Part print with two shaded views. Sizes in mm from the minimum x, y, z corner. Coordinates: 2 decimals unless noted, no trailing zeros. Write each loop counter-clockwise with the first axis right and the second up, starting at its lowest first coordinate (ties: lowest second). Pieces come first, ordered by that corner, then holes.
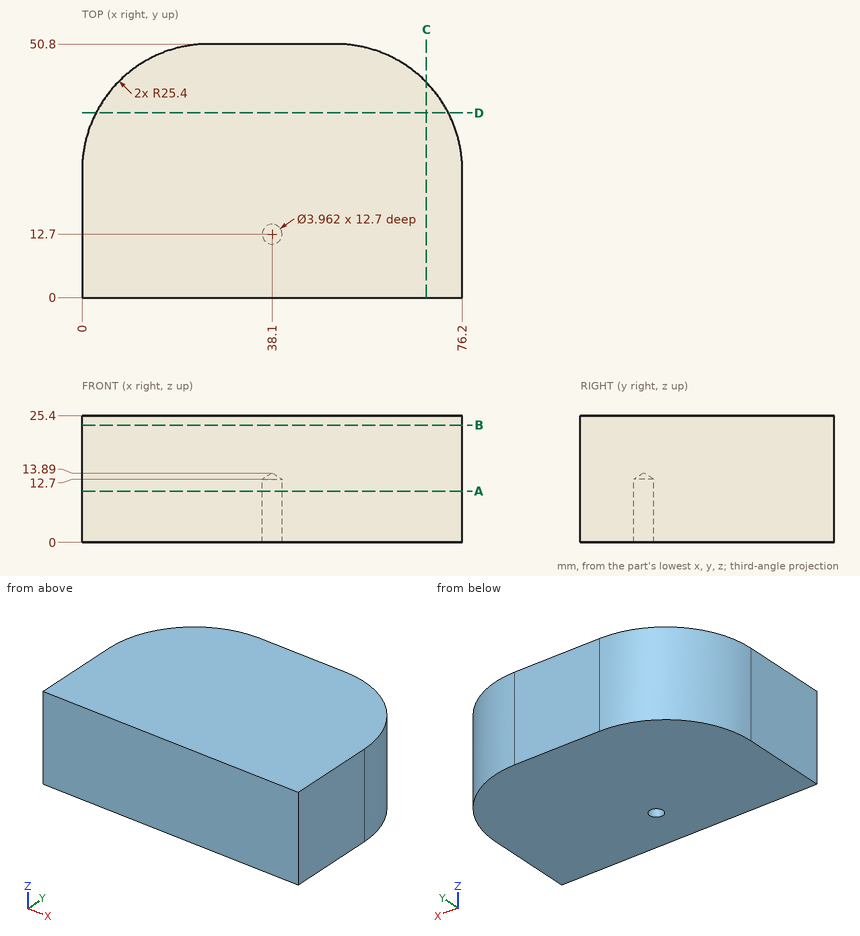
(1) Slice it at D-D, the plane y = 37. List the corners of the cut face in (x, z), and give its area (3 significant figures).
(2) Slice it at B-B, the plane z = 23.5. List the corners of the cut face in (x, y), and give its area (3 significant figures).
(3) Probe L1, parallel to X at y = 12.5, z = 8; L2, parallel to Y at x = 38.1, z = 6.75; L3, parallel to Y at x = 51, z = 15. List the from-to ranges inside material, lowest first.
(4) Slice it at C-C, the plane x = 69. List the corners of the cut face in (y, z).
(5) Slice it at A-A, the plane z = 10.25. List the corners of the cut face in (x, y).
(6) Flat gauge pins, fed straight in: P1, Ø2, axis at y = 44.5, z = 6.5, coming from the +X side; P2, Ø6, axis at y = 33, z = 16.5, coming from the +X side; P3, Ø3, axis at x = 38.1, y = 12.7, coming from the -Z side. Where does each tip first touch, or does it go through?
Results:
1. outline: (2.8, 0) - (73.4, 0) - (73.4, 25.4) - (2.8, 25.4) - close
1. area: 1,790 mm2
2. outline: (0, 0) - (76.2, 0) - (76.2, 25.4) arc R25.4 ccw to (50.8, 50.8) - (25.4, 50.8) arc R25.4 ccw to (0, 25.4) - close
2. area: 3,590 mm2
3. L1: x = 0 to 36.13, 40.07 to 76.2
3. L2: y = 0 to 10.72, 14.68 to 50.8
3. L3: y = 0 to 50.8
4. outline: (0, 0) - (43.12, 0) - (43.12, 25.4) - (0, 25.4) - close
5. outline: (0, 0) - (76.2, 0) - (76.2, 25.4) arc R25.4 ccw to (50.8, 50.8) - (25.4, 50.8) arc R25.4 ccw to (0, 25.4) - close; hole circle Ø3.96 at (38.1, 12.7)
6. P1: stops at x = 68.62
6. P2: stops at x = 75.78
6. P3: stops at z = 12.99
